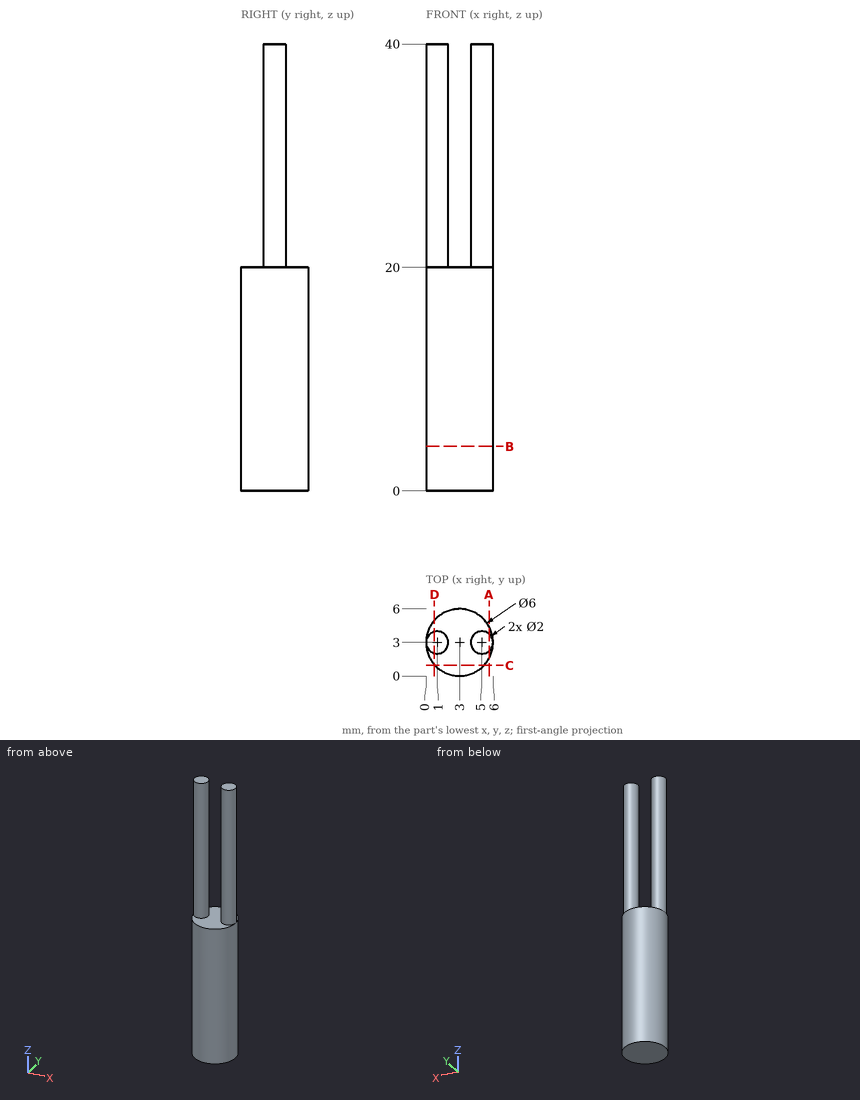
Check sheet for the drawn part. Datum: minimum x, y, z corner. Units: mm. Give positions to 0.01 mm unless a question says otherwise; leave off trailing zeros. Order: outer loops, then holes, each group sorted by start corner. A loop starts at its lowest first (then second) coordinate and runs counter-clockwise, first axis right, second up. Notation, with made-up numbers: (30, -4) - (87, -4) arc R21 ccw to (87, 20) - close; hole circle Ø7 at (49.25, 55). An arc over 180 degrees is marked (long way). Answer as a JSON object with one key per item and string values.
(1) Depth check by flat-ended pin: pin 1 Ø3 at (x, y) = (2.5, 5.5) entering from +Z. Enter the tip coordinate at first touch or a pass-through.
Report:
{"pin 1": "z = 20"}
(2) Cross-section at D-D (x = 0.75). Record the cut outline in (y, z), then the cut area to 3 significant figures.
Report:
{"outline": "(1.02, 0) - (4.98, 0) - (4.98, 20) - (3.97, 20) - (3.97, 40) - (2.03, 40) - (2.03, 20) - (1.02, 20) - close", "area": "118 mm^2"}
(3) Cross-section at B-B (z = 4). Record the cut outline in (x, y), then the cut area to 3 significant figures.
Report:
{"outline": "circle Ø6 at (3, 3)", "area": "28.3 mm^2"}
(4) Material ranges on line 1 (Y direction, x = 5, z = 21); line 2 (Z direction, x = 1.85, y = 5.1); line 3 (X direction, y = 3.3, z = 37), recorded low to high.
Report:
{"line 1": "2 to 4", "line 2": "0 to 20", "line 3": "0.05 to 1.95, 4.05 to 5.95"}
(5) Cross-section at C-C (y = 0.95). Record the cut outline in (x, z), then the cut area to 3 significant figures.
Report:
{"outline": "(0.81, 0) - (5.19, 0) - (5.19, 20) - (0.81, 20) - close", "area": "87.6 mm^2"}
(6) Cross-section at A-A (x = 5.65). Record the cut outline in (y, z).
Report:
{"outline": "(1.59, 0) - (4.41, 0) - (4.41, 20) - (3.76, 20) - (3.76, 40) - (2.24, 40) - (2.24, 20) - (1.59, 20) - close"}
